For this review, take the finished solid that the model builds, in its own axes (mm). A direction names the side the tool comes from. Coordinates: 2 decimals unless noted, no trailing zeros. Order: outer loops, then holes, each group sorted by start corner. A loop starts at its lowest first (then second) coordinate and runs counter-clockwise, first axis right, second up. Notation, with made-up numbers: M 59.25,84 L 115.25,84 A26 cw 115.25,106 Z; hole C 40,-39.75 d5. An arc over 180 degrees is marked long. Use CSV: the item, a comma, the result in double quotes.
```python
from build123d import *

# Parameters (mm, degrees)
SKETCH1_W                   = 11.5
SKETCH1_H                   = 22.5
PCB_DEPTH                   = 1.5
SKETCH2_4_R                 = 0.6
INITIAL_INPUT_HOLES_DEPTH   = 13.72301065
INPUT_HOLES_LPATTERN_COUNT  = 4
INPUT_HOLES_LPATTERN_PITCH  = 2.5
SKETCH2_3_R                 = 0.6
INITIAL_OUTPUT_HOLE_DEPTH   = 13.72301065
OUTPUT_HOLES_LPATTERN_COUNT = 2
OUTPUT_HOLES_LPATTERN_PITCH = 3
SKETCH2_R                   = 1.25
MOUNTING_HOLES_DEPTH        = 13.72301065
SKETCH3_4_W                 = 1.3
SKETCH3_4_H                 = 2.15
CAPACITORS_DEPTH            = 0.55
SKETCH3_3_W                 = 1.25
SKETCH3_3_H                 = 2.15
RESISTORS_DEPTH             = 0.45
SKETCH3_W                   = 5
SKETCH3_H                   = 3.85
TRANSCEIVER_CHIP_DEPTH      = 1.5


with BuildPart() as part:
    # Sketch1 → PCB (new body)
    with BuildSketch(Plane(origin=(0, 0, 0), x_dir=(1, 0, 0), z_dir=(0, 1, 0))):
        Rectangle(SKETCH1_W, SKETCH1_H)
    extrude(amount=PCB_DEPTH)

    # Sketch2_4 → Initial Input Holes (cut, through all)
    with BuildSketch(Plane(origin=(0, 1.5, 0), x_dir=(1, 0, 0), z_dir=(0, 1, 0))):
        with Locations(Location((-3.75, -9.9, 0), (0, 0, 270))):
            Circle(SKETCH2_4_R)
    initial_input_holes = extrude(amount=-INITIAL_INPUT_HOLES_DEPTH, mode=Mode.SUBTRACT)

    # Input Holes LPattern: Initial Input Holes ×4
    with Locations(*[(i * INPUT_HOLES_LPATTERN_PITCH, 0, 0) for i in range(1, INPUT_HOLES_LPATTERN_COUNT)]):
        add(initial_input_holes, mode=Mode.SUBTRACT)

    # Sketch2_3 → Initial Output Hole (cut, through all)
    with BuildSketch(Plane(origin=(0, 1.5, 0), x_dir=(1, 0, 0), z_dir=(0, 1, 0))):
        with Locations(Location((-1.75, 9.75, 0), (0, 0, 270))):
            Circle(SKETCH2_3_R)
    initial_output_hole = extrude(amount=-INITIAL_OUTPUT_HOLE_DEPTH, mode=Mode.SUBTRACT)

    # Output Holes LPattern: Initial Output Hole ×2
    with Locations(*[(i * OUTPUT_HOLES_LPATTERN_PITCH, 0, 0) for i in range(1, OUTPUT_HOLES_LPATTERN_COUNT)]):
        add(initial_output_hole, mode=Mode.SUBTRACT)

    # Sketch2 → Mounting Holes (cut, through all)
    with BuildSketch(Plane(origin=(0, 1.5, 0), x_dir=(1, 0, 0), z_dir=(0, 1, 0))):
        with Locations(Location((-4.25, 9.75, 0), (0, 0, 270))):
            Circle(SKETCH2_R)
        with Locations(Location((4.25, 9.75, 0), (0, 0, 270))):
            Circle(SKETCH2_R)
    extrude(amount=-MOUNTING_HOLES_DEPTH, mode=Mode.SUBTRACT)

    # Sketch3_4 → Capacitors (add)
    with BuildSketch(Plane(origin=(0, 1.5, 0), x_dir=(1, 0, 0), z_dir=(0, 1, 0))):
        with Locations((2, 2.925)):
            Rectangle(SKETCH3_4_W, SKETCH3_4_H)
        with Locations((4.6, 2.925)):
            Rectangle(SKETCH3_4_W, SKETCH3_4_H)
        with Locations((-4.1, -4.775)):
            Rectangle(SKETCH3_4_W, SKETCH3_4_H)
    extrude(amount=CAPACITORS_DEPTH)

    # Sketch3_3 → Resistors (add)
    with BuildSketch(Plane(origin=(0, 1.5, 0), x_dir=(1, 0, 0), z_dir=(0, 1, 0))):
        with Locations((-1.525, -4.775)):
            Rectangle(SKETCH3_3_W, SKETCH3_3_H)
        with Locations((1.055, -4.775)):
            Rectangle(SKETCH3_3_W, SKETCH3_3_H)
        with Locations((4.155, -4.775)):
            Rectangle(SKETCH3_3_W, SKETCH3_3_H)
    extrude(amount=RESISTORS_DEPTH)

    # Sketch3 → Transceiver Chip (add)
    with BuildSketch(Plane(origin=(0, 1.5, 0), x_dir=(1, 0, 0), z_dir=(0, 1, 0))):
        with Locations((-2.9, 3.825)):
            Rectangle(SKETCH3_W, SKETCH3_H)
    extrude(amount=TRANSCEIVER_CHIP_DEPTH)


solid = part.part
```
Item 1: To check wall thickness, follow line 1 along X through (y, z) = (1.9, 5.25); line 2 along X through (y, z) = (0.5, -9.75); line 3 along X through (y, z) = (0.7, 9.9). State the ranges of each line that lie inside material, in increasing order. Write a range as [from, to].
Solutions:
line 1,"[-4.75, -3.45], [-2.15, -0.9], [0.43, 1.68], [3.53, 4.78]"
line 2,"[-5.75, -5.5], [-3, -2.35], [-1.15, 0.65], [1.85, 3], [5.5, 5.75]"
line 3,"[-5.75, -4.35], [-3.15, -1.85], [-0.65, 0.65], [1.85, 3.15], [4.35, 5.75]"
Item 2: Draft analysis for pull direction X (two halves, no side actions). For faces 1 (the face through (-5.01, 0.76, -10.74)), 2 (the face through (5.75, 1, 0)), 3 (the face through (-1.5, 1.95, 4.8)), state which applies: released by +X, released by -X, zero draft, split by the parting line, or undercut.
Solutions:
face 1,"undercut"
face 2,"released by +X"
face 3,"zero draft"
Item 3: Add section A-A on z = 9.9. State the section outline as (x, y) points.
Solutions:
outline,"M -5.75,0 L -4.35,0 L -4.35,1.5 L -5.75,1.5 Z; M -3.15,0 L -1.85,0 L -1.85,1.5 L -3.15,1.5 Z; M -0.65,0 L 0.65,0 L 0.65,1.5 L -0.65,1.5 Z; M 1.85,0 L 3.15,0 L 3.15,1.5 L 1.85,1.5 Z; M 4.35,0 L 5.75,0 L 5.75,1.5 L 4.35,1.5 Z"
Item 4: Clearance check with flat-ended pins moving along their axes: pin 1 Ø1.4 at (x, z) = (1.25, 9.9) entering from -Y; pin 2 Ø1.1 at (x, z) = (1.25, -9.75) entering from -Y; pin 3 Ø0.6 at (y, z) = (2, -2.5) entering from -X; pin 4 Ø1.6 at (x, z) = (3.75, 9.9) entering from +Y. State where each tip first meets the part, or that it passes through.
Solutions:
pin 1,"y = 0"
pin 2,"through"
pin 3,"x = -5.4"
pin 4,"y = 1.5"
Item 5: For faces 4 (the face through (3.78, 0.76, 9.3)), 5 (the face through (-4, 2.05, 5)), 6 (the face through (-3, 2, -5.75)), 7 (the face through (-0.4, 2, -4)), 8 (the face through (2, 2.05, -3)), list the 3-axis set-ups (+Z, -Z, +X, -X, +Y, -Y) from which the entire face can be reached by the end or side of a thin tool; tool diameter is ignored.
Solutions:
face 4,"+Y, -Y"
face 5,"+Z, +X, -X, +Y"
face 6,"-Z, +X, -X, +Y"
face 7,"+Z, -Z, +Y"
face 8,"+Z, -Z, +X, +Y"
Item 6: Add section D-D on z = 6.75. State the section outline as (x, y) points.
Solutions:
outline,"M -5.75,0 L 5.75,0 L 5.75,1.5 L -5.75,1.5 Z"
Item 7: Add section C-C on z = -9.75. State the section outline as (x, y) points, and give its area (3 significant figures).
Solutions:
outline,"M -5.75,0 L -5.5,0 L -5.5,1.5 L -5.75,1.5 Z; M -3,0 L -2.35,0 L -2.35,1.5 L -3,1.5 Z; M -1.15,0 L 0.65,0 L 0.65,1.5 L -1.15,1.5 Z; M 1.85,0 L 3,0 L 3,1.5 L 1.85,1.5 Z; M 5.5,0 L 5.75,0 L 5.75,1.5 L 5.5,1.5 Z"
area,"6.15 mm^2"
Item 8: Add section B-B on x = 0. State the section outline as (y, z) points.
Solutions:
outline,"M 0,-11.25 L 1.5,-11.25 L 1.5,11.25 L 0,11.25 Z"
